Geometry: final body of the model. Coordinates: model frame, mm. A direction names the side the tool comes from. Coordinates: 2 decimals unless noted, no trailing zeros. Order: outer loops, then holes, each group sorted by start corner. A loop starts at its lowest first (then second) coordinate and runs counter-clockwise, first axis right, second up. Notation, with made-up numbers: M 34.25,13.5 L 42.25,13.5 A26 cw 42.25,50.5 Z; hole C -27,-2 d7. An arc over 180 degrees is marked long. Use CSV: the item, a comma, the result in double quotes. Start each with the question number.
1. Section query D-D on x = 1083. Return the cut outline in (y, z), and give its area (3 significant figures).
2. Section query B-B on y = -177.5. Return the cut outline in (x, z).
3. Section query A-A on y = 0. Return the cut outline in (x, z).
4. Pull-direction query (X, two-part tool) for faces 4 (the cylindrical face through (258.28, -214.61, -67.58)), 5 (the flat face through (156.301, -103, -53)), 6 (the flat face through (799, 76.829, 1)); classes: pulls with the +X half, pulls with the -X half, needs draft (parallel to the pull), parting line crosses it, or undercut.
5. Set-up query: faces 1 (the flat face through (923, -66.829, -1)), 2 (the flat face through (1063.776, -91, 1)), 3 (the flat face through (923, 66.829, -1)). Return all of +Z, -Z, +X, -X, +Y, -Y with unobstructed straight access to the full face (end or side cutting, diameter ignored); none if empty.
6. First-contact query: P1, Ø10, axis at x = 1531, y = -117, coming from the -Z side; P2, Ø11, axis at y = -88.5, z = -38.5, coming from the -X side; P3, Ø12, axis at x = 1639.5, y = -137.5, coming from the -Z side; P4, Ø1, axis at y = -23, z = 126.5, coming from the +X side. Flat tips, straight axial feed; report the tip coordinate or a pass-through.
7. Material intervals for line 1 (X direction, y = -82.5, z = -98); line 2 (Z direction, x = 1009, y = -8.5); line 3 (Z direction, x = 1262, y = 25.5), sorted ascending.
8. Section query C-C on x = 1622. Return the cut outline in (y, z), and give its area (3 significant figures).
from build123d import *

# Parameters (mm, degrees)
SKETCH2_W          = 277.551020408
SKETCH2_H          = 73.171214091
CUT_EXTRUDE1_DEPTH = 1896.296810529
SKETCH3_R          = 125
CUT_EXTRUDE2_DEPTH = 10


with BuildPart() as part:
    # Sketch1 → Revolve1 (revolve)
    with BuildSketch(Plane.XY, mode=Mode.PRIVATE) as revolve1_sk:
        Polygon((0, 0), (0, 113.414392954), (156.301438496, 113.414392954), (156.301438496, 225), (357.44745317, 225), (357.44745317, 113.414392954), (1492.55254683, 113.414392954), (1492.55254683, 225), (1693.698561504, 225), (1693.698561504, 113.414392954), (1850, 113.414392954), (1850, 0), align=None)
    revolve(revolve1_sk.sketch.rotate(Axis((0, 0, 0), (1, 0, 0)), 180), axis=Axis((0, 0, 0), (1, 0, 0)))

    # Sketch2 → Cut-Extrude1 (cut, through all)
    with BuildSketch(Plane.XY.offset(120)):
        with Locations((925, 113.414392955)):
            Rectangle(SKETCH2_W, SKETCH2_H)
        with Locations((925, -113.414392955)):
            Rectangle(SKETCH2_W, SKETCH2_H)
    extrude(amount=-CUT_EXTRUDE1_DEPTH, mode=Mode.SUBTRACT)

    # Sketch3 → Cut-Extrude2 (cut)
    with BuildSketch(Plane(origin=(0, 76.828785909, 0), x_dir=(1, 0, 0), z_dir=(0, 1, 0))):
        with Locations((925, 0)):
            Circle(SKETCH3_R)
    cut_extrude2 = extrude(amount=-CUT_EXTRUDE2_DEPTH, mode=Mode.SUBTRACT)

    # Mirror1: Cut-Extrude2 across plane
    add(cut_extrude2.mirror(Plane.ZX), mode=Mode.SUBTRACT)


solid = part.part
Results list:
1,outline,"C 0,0 d226.83"
1,area,"40,400 mm²"
2,outline,"M 156.3,-138.27 L 357.45,-138.27 L 357.45,138.27 L 156.3,138.27 Z; M 1492.55,-138.27 L 1693.7,-138.27 L 1693.7,138.27 L 1492.55,138.27 Z"
3,outline,"M 0,-113.41 L 156.3,-113.41 L 156.3,-225 L 357.45,-225 L 357.45,-113.41 L 1492.55,-113.41 L 1492.55,-225 L 1693.7,-225 L 1693.7,-113.41 L 1850,-113.41 L 1850,113.41 L 1693.7,113.41 L 1693.7,225 L 1492.55,225 L 1492.55,113.41 L 357.45,113.41 L 357.45,225 L 156.3,225 L 156.3,113.41 L 0,113.41 Z"
4,face 4,"needs draft"
4,face 5,"pulls with the -X half"
4,face 6,"undercut"
5,face 1,"-Y"
5,face 2,"+Z, -Z, -Y"
5,face 3,"+Y"
6,P1,"stops at z = -195.14"
6,P2,"stops at x = 0"
6,P3,"stops at z = -182.57"
6,P4,"stops at x = 1693.7"
7,line 1,"x = 156.3 to 357.45, 1492.55 to 1693.7"
7,line 2,"z = -113.1 to 113.1"
7,line 3,"z = -110.51 to 110.51"
8,outline,"C 0,0 d450"
8,area,"159,000 mm²"
